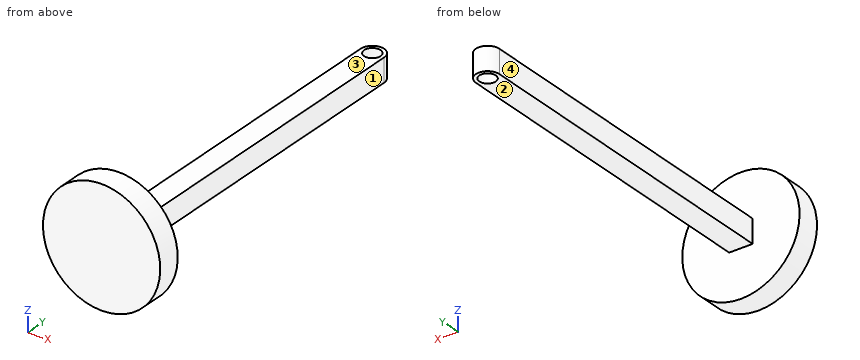
```python
from build123d import *

# Parameters (mm, degrees)
SKETCH1_R           = 3.5
BOSS_EXTRUDE1_DEPTH = 10
SKETCH2_R           = 25
BOSS_EXTRUDE2_DEPTH = 5


with BuildPart() as part:
    # Sketch1 → Boss-Extrude1 (new body)
    with BuildSketch(Plane.XY):
        with BuildLine():
            Line((-5, 0), (-5, -150))
            Line((-5, -150), (5, -150))
            Line((5, -150), (5, 0))
            ThreePointArc((5, 0), (0, 5), (-5, 0))
        make_face()
        Circle(SKETCH1_R, mode=Mode.SUBTRACT)
    extrude(amount=BOSS_EXTRUDE1_DEPTH)

    # Sketch2 → Boss-Extrude2 (add, symmetric)
    with BuildSketch(Plane.XZ.offset(150)):
        with Locations(Location((0, 5, 0), (0, 0, 270))):
            Circle(SKETCH2_R)
    extrude(amount=BOSS_EXTRUDE2_DEPTH, both=True)


solid = part.part
```
Can you work these out from the model? Positions are in its coordinate system, mm. Face numbers are marked on the shaded views. A direction names the side the tool comes from. Give positions to 0.01 mm unless a question says otherwise; leave off trailing zeros. Order: outer loops, then holes, each group sorted by start corner. A loop starts at its lowest first (then second) coordinate and runs counter-clockwise, first axis right, second up. Notation, with made-up numbers: (24.25, 1) - (52.25, 1) arc R14 cw to (52.25, 18) - close; hole circle Ø3 at (-26, -7.5). An arc over 180 degrees is marked (long way). Use a Markdown table: item, result. Add a question column.
Q1. If we section it at B-B on z = 5: Write out the boundary of the cut face in (x, y).
Q2. I'm going to push flat-ended pins straight in: pin 1 (3 mm diameter, centred on y = -59.5, z = 3.5, fed in from -X); pin 2 (3 mm diameter, centred on x = -1, y = -35.5, fed in from -Z); pin 3 (12 mm diameter, centred on x = 12, y = -121, fed in from -Z); pin 4 (8 mm diameter, centred on x = -0.5, y = -89, fed in from +Z). Where does each tip first touch, or does it pass through?
Q3. If we section it at C-C on y = -36.5: Write out the boundary of the cut face in (x, z).
Q4. Please list where these lines run through material, in increasing order: line 1 along Y through (x, z) = (0, 6); line 2 along Z through (x, y) = (1, -79.5); line 3 along Y through (x, z) = (15.5, 13).
Q5. On a 3-axis mill with a long thin cutter (end or side, diameter ignored), from which of +Z, -Z, +X, -X, +Y, -Y can I reach the whole of each face in a straight line? I mean the marked faces 1, 2, 3 and 4. Say none if no direction works.
Q6. If we section it at D-D on z = 12: Write out the boundary of the cut face in (x, y).
Q7. If we section it at A-A on x = 0: Write out the boundary of the cut face in (y, z).
Answers follow:
| question | item | result |
|---|---|---|
| 1 | outline | (-25, -155) - (25, -155) - (25, -145) - (5, -145) - (5, 0) arc R5 ccw to (-5, 0) - (-5, -145) - (-25, -145) - close; hole circle Ø7 at (0, 0) |
| 2 | pin 1 | stops at x = -5 |
| 2 | pin 2 | stops at z = 0 |
| 2 | pin 3 | passes through |
| 2 | pin 4 | stops at z = 10 |
| 3 | outline | (-5, 0) - (5, 0) - (5, 10) - (-5, 10) - close |
| 4 | line 1 | y = -155 to -3.5, 3.5 to 5 |
| 4 | line 2 | z = 0 to 10 |
| 4 | line 3 | y = -155 to -145 |
| 5 | face 1 | +Z, -Z, +X, +Y |
| 5 | face 2 | -Z, +X, -X, +Y |
| 5 | face 3 | +Z, +X, -X, +Y |
| 5 | face 4 | +Z, -Z, -X, +Y |
| 6 | outline | (-24, -155) - (24, -155) - (24, -145) - (-24, -145) - close |
| 7 | outline | (-155, -20) - (-145, -20) - (-145, 0) - (-3.5, 0) - (-3.5, 10) - (-145, 10) - (-145, 30) - (-155, 30) - close; (3.5, 0) - (5, 0) - (5, 10) - (3.5, 10) - close |
